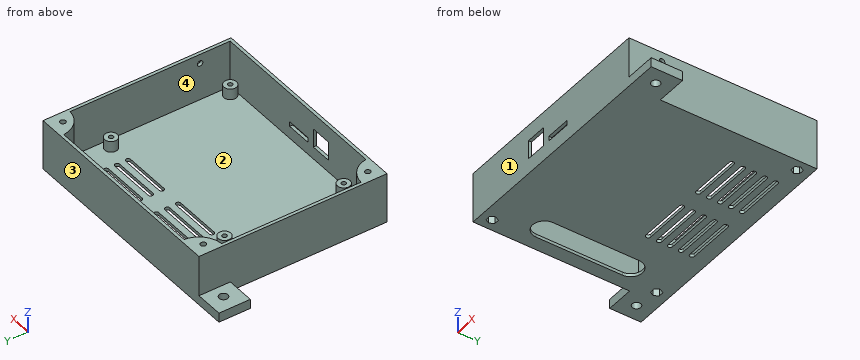
from build123d import *

# Parameters (mm, degrees)
SKETCH_W        = 140
SKETCH_H        = 120
PAD_DEPTH       = 32
THICKNESS_T     = -2
SKETCH001_R     = 4
SKETCH001_R_2   = 1.45
PAD001_DEPTH    = 7
SKETCH002_W     = 16.413659
SKETCH002_H     = 3.088
SKETCH002_W_2   = 13.5
SKETCH002_H_2   = 12
POCKET_DEPTH    = 44.151
PAD002_DEPTH    = 32
SKETCH004_R     = 1.75
POCKET001_DEPTH = 58.836
SKETCH005_R     = 1.75
POCKET002_DEPTH = 32.001001
SKETCH006_W     = 20
SKETCH006_H     = 20
SKETCH006_R     = 2.75
PAD003_DEPTH    = 6
POCKET003_DEPTH = 29
POCKET004_DEPTH = 32.001001


with BuildPart() as part:
    # Sketch → Pad (new body)
    with BuildSketch(Plane.XY):
        with Locations((-11.165, 15.85)):
            Rectangle(SKETCH_W, SKETCH_H)
    extrude(amount=PAD_DEPTH)

    # Thickness
    thickness_openings = [part.faces().sort_by_distance(p)[0] for p in [
        (-11.165, 15.85, 32),
    ]]
    offset(amount=THICKNESS_T, openings=thickness_openings, kind=Kind.INTERSECTION)

    # Sketch001 (on DatumPlane) → Pad001 (join)
    with BuildSketch(Plane.XY.offset(2)):
        with Locations((-50.925, 38.05)):
            Circle(SKETCH001_R)
        with Locations((-50.925, 38.05)):
            Circle(SKETCH001_R_2, mode=Mode.SUBTRACT)
        with Locations((50.925, 38.05)):
            Circle(SKETCH001_R)
        with Locations((50.925, 38.05)):
            Circle(SKETCH001_R_2, mode=Mode.SUBTRACT)
        with Locations((-50.925, -38.05)):
            Circle(SKETCH001_R)
        with Locations((-50.925, -38.05)):
            Circle(SKETCH001_R_2, mode=Mode.SUBTRACT)
        with Locations((50.925, -38.05)):
            Circle(SKETCH001_R)
        with Locations((50.925, -38.05)):
            Circle(SKETCH001_R_2, mode=Mode.SUBTRACT)
    extrude(amount=PAD001_DEPTH)

    # Sketch002 → Pocket (cut, through all)
    with BuildSketch(Plane.XZ):
        with Locations((-4.884073, 11.44743)):
            Rectangle(SKETCH002_W, SKETCH002_H)
        with Locations((-24.636516, 15.847709)):
            Rectangle(SKETCH002_W_2, SKETCH002_H_2)
    extrude(amount=POCKET_DEPTH, mode=Mode.SUBTRACT)

    # Sketch003 → Pad002 (join)
    with BuildSketch(Plane.XY):
        with BuildLine():
            Line((43, 75), (58, 75))
            Line((58, 75), (58, 60))
            ThreePointArc((43, 75), (47.393398, 64.393398), (58, 60))
        make_face()
        with BuildLine():
            Line((-80, 75), (-65, 75))
            ThreePointArc((-80, 60), (-69.393398, 64.393398), (-65, 75))
            Line((-80, 75), (-80, 60))
        make_face()
        with BuildLine():
            Line((-80, -29), (-80, -44))
            Line((-80, -44), (-65, -44))
            ThreePointArc((-65, -44), (-69.393398, -33.393398), (-80, -29))
        make_face()
    extrude(amount=PAD002_DEPTH)

    # Sketch004 → Pocket001 (cut, through all)
    with BuildSketch(Plane.YZ):
        with Locations((-23, 26)):
            Circle(SKETCH004_R)
    extrude(amount=POCKET001_DEPTH, mode=Mode.SUBTRACT)

    # Sketch005 → Pocket002 (cut, through all)
    with BuildSketch(Plane.XY):
        with Locations((-74, 68)):
            Circle(SKETCH005_R)
        with Locations((52, 68)):
            Circle(SKETCH005_R)
        with Locations((-74, -37)):
            Circle(SKETCH005_R)
    extrude(amount=POCKET002_DEPTH, mode=Mode.SUBTRACT)

    # Sketch006 → Pad003 (join)
    with BuildSketch(Plane.XY):
        with Locations((68.8, -34.15)):
            Rectangle(SKETCH006_W, SKETCH006_H)
        with Locations((68.8, -34.15)):
            Circle(SKETCH006_R, mode=Mode.SUBTRACT)
        with Locations((-89.1, 65.85)):
            Rectangle(SKETCH006_W, SKETCH006_H)
        with Locations((-89.1, 65.85)):
            Circle(SKETCH006_R, mode=Mode.SUBTRACT)
    extrude(amount=PAD003_DEPTH)

    # Sketch007 → Pocket003 (cut)
    with BuildSketch(Plane.XY):
        Polygon((-70.75, 68), (-72.375, 70.814583), (-75.625, 70.814583), (-77.25, 68), (-75.625, 65.185417), (-72.375, 65.185417), align=None)
        Polygon((55.25, 68), (53.625, 70.814583), (50.375, 70.814583), (48.75, 68), (50.375, 65.185417), (53.625, 65.185417), align=None)
        Polygon((-70.75, -37), (-72.375, -34.185417), (-75.625, -34.185417), (-77.25, -37), (-75.625, -39.814583), (-72.375, -39.814583), align=None)
    extrude(amount=POCKET003_DEPTH, mode=Mode.SUBTRACT)

    # Sketch008 → Pocket004 (cut, through all)
    with BuildSketch(Plane.XY):
        with BuildLine():
            ThreePointArc((-57.5, 45), (-65, 52.5), (-72.5, 45))
            Line((-72.5, 45), (-72.5, -10))
            ThreePointArc((-72.5, -10), (-65, -17.5), (-57.5, -10))
            Line((-57.5, -10), (-57.5, 45))
        make_face()
        with BuildLine():
            ThreePointArc((7, 66.5), (5.5, 65), (7, 63.5))
            Line((7, 63.5), (37, 63.5))
            ThreePointArc((37, 63.5), (38.5, 65), (37, 66.5))
            Line((37, 66.5), (7, 66.5))
        make_face()
        with BuildLine():
            ThreePointArc((-38, 66.5), (-39.5, 65), (-38, 63.5))
            Line((-38, 63.5), (-8, 63.5))
            ThreePointArc((-8, 63.5), (-6.5, 65), (-8, 66.5))
            Line((-8, 66.5), (-38, 66.5))
        make_face()
        with BuildLine():
            ThreePointArc((-38, 59.5), (-39.5, 58), (-38, 56.5))
            Line((-38, 56.5), (-8, 56.5))
            ThreePointArc((-8, 56.5), (-6.5, 58), (-8, 59.5))
            Line((-8, 59.5), (-38, 59.5))
        make_face()
        with BuildLine():
            ThreePointArc((7, 59.5), (5.5, 58), (7, 56.5))
            Line((7, 56.5), (37, 56.5))
            ThreePointArc((37, 56.5), (38.5, 58), (37, 59.5))
            Line((37, 59.5), (7, 59.5))
        make_face()
        with BuildLine():
            ThreePointArc((-38, 52.5), (-39.5, 51), (-38, 49.5))
            Line((-38, 49.5), (-8, 49.5))
            ThreePointArc((-8, 49.5), (-6.5, 51), (-8, 52.5))
            Line((-8, 52.5), (-38, 52.5))
        make_face()
        with BuildLine():
            ThreePointArc((7, 52.5), (5.5, 51), (7, 49.5))
            Line((7, 49.5), (37, 49.5))
            ThreePointArc((37, 49.5), (38.5, 51), (37, 52.5))
            Line((37, 52.5), (7, 52.5))
        make_face()
        with BuildLine():
            ThreePointArc((-38, 45.5), (-39.5, 44), (-38, 42.5))
            Line((-38, 42.5), (-8, 42.5))
            ThreePointArc((-8, 42.5), (-6.5, 44), (-8, 45.5))
            Line((-8, 45.5), (-38, 45.5))
        make_face()
        with BuildLine():
            ThreePointArc((7, 45.5), (5.5, 44), (7, 42.5))
            Line((7, 42.5), (37, 42.5))
            ThreePointArc((37, 42.5), (38.5, 44), (37, 45.5))
            Line((37, 45.5), (7, 45.5))
        make_face()
        with BuildLine():
            ThreePointArc((-38, 38.5), (-39.5, 37), (-38, 35.5))
            Line((-38, 35.5), (-8, 35.5))
            ThreePointArc((-8, 35.5), (-6.5, 37), (-8, 38.5))
            Line((-8, 38.5), (-38, 38.5))
        make_face()
        with BuildLine():
            ThreePointArc((7, 38.5), (5.5, 37), (7, 35.5))
            Line((7, 35.5), (37, 35.5))
            ThreePointArc((37, 35.5), (38.5, 37), (37, 38.5))
            Line((37, 38.5), (7, 38.5))
        make_face()
    extrude(amount=POCKET004_DEPTH, mode=Mode.SUBTRACT)


solid = part.part
Part model, mm, in its own coordinate system. Face numbers are marked on the shaded views. A direction names the side the tool comes from. Give positions to 0.01 mm unless a question says otherwise; leave off trailing zeros. Loops run counter-clockwise (first coordinate to the right, second up) from the corner with the lowest first, then second, coordinate; pieces in that order, holes last. Notation, with made-up numbers: (-26, 43) -> (27, 43) arc R13 cw to (27, 62) -> close; hole circle Ø3 at (46, 22). An arc over 180 degrees is marked (long way). Write each question's results on one line, items separated by ' | '. Start each with the question number.
Q1. Which spindle directions (+Z, -Z, +X, -X, +Y, -Y) get a long thin tool onto all of the face, cutting with end or side? Do the marked faces 1 and 2. Say none if no direction does.
Q2. Wall check: L1, parallel to Y at x = 57, z = 26; L2, parallel to Y at x = -2.5, z = 3; L3, parallel to X at y = 50.5, z = 3 (3 decimals). Give the ranges that are in metal, low to high.
Q3. Band-saw the part on D-D on x = -41.5. List the corners of the cut face in (y, z), plus the area to 3 significant figures.
Q4. Pull direction X, two halves, no side cores. Call the marked faces 3 and 4: +X half, -X half, draft (parallel to the pull), parting line (faces both ways), or undercut.
Q5. Pin check, flat tips, straight feed: P1, Ø3, axis at x = -90.5, z = 2.5, coming from the -Y side; P2, Ø10, axis at x = 45.5, y = -25.5, coming from the +Z side; P3, Ø1, axis at x = -37.5, y = 41.5, coming from the -Z side; P4, Ø0.6, axis at y = -43.5, z = 18, coming from the -X side (3 decimals). Stop position of each tip, or through.
Q6. Band-saw the part on C-C on z = 17. Count the separate pieces of the cut face and the enclosed holes in it, plus the area to 3 significant figures.
Q7. Band-saw the part on B-B on y = 2. List the corners of the cut face in (x, z) (3 decimals).
Q8. Band-saw the part on A-A on x = 25. List the corners of the cut face in (y, z).
Results are:
1) face 1: +Z, -Z, +X, -X, -Y | face 2: +Z
2) L1: y = -44.15 to -24.75, -21.25 to 75.85 | L2: y = -44.15 to -42.15, 73.85 to 75.85 | L3: x = -81.165 to -79.165, 56.835 to 58.835
3) outline: (-44.15, 0) -> (75.85, 0) -> (75.85, 32) -> (73.85, 32) -> (73.85, 2) -> (-42.15, 2) -> (-42.15, 32) -> (-44.15, 32) -> close | area: 360 mm²
4) face 3: draft | face 4: undercut
5) P1: stops at y = 55.85 | P2: stops at z = 2 | P3: stops at z = 0 | P4: stops at x = -81.165
6) separate pieces: 1 | enclosed holes: 3 | area: 1,340 mm²
7) outline: (-81.165, 0) -> (-72.5, 0) -> (-72.5, 2) -> (-79.165, 2) -> (-79.165, 32) -> (-81.165, 32) -> close; (-57.5, 0) -> (58.835, 0) -> (58.835, 32) -> (56.835, 32) -> (56.835, 2) -> (-57.5, 2) -> close
8) outline: (-44.15, 0) -> (35.5, 0) -> (35.5, 2) -> (-42.15, 2) -> (-42.15, 32) -> (-44.15, 32) -> close; (38.5, 0) -> (42.5, 0) -> (42.5, 2) -> (38.5, 2) -> close; (45.5, 0) -> (49.5, 0) -> (49.5, 2) -> (45.5, 2) -> close; (52.5, 0) -> (56.5, 0) -> (56.5, 2) -> (52.5, 2) -> close; (59.5, 0) -> (63.5, 0) -> (63.5, 2) -> (59.5, 2) -> close; (66.5, 0) -> (75.85, 0) -> (75.85, 32) -> (73.85, 32) -> (73.85, 2) -> (66.5, 2) -> close
